from build123d import *

# Parameters (mm, degrees)
BOSS_EXTRUDE1_DEPTH   = 2
F_4_0MM_DOWEL_HOLE1_D = 4


with BuildPart() as part:
    # Sketch1 → Boss-Extrude1 (new body)
    with BuildSketch(Plane(origin=(0, 0, 0), x_dir=(1, 0, 0), z_dir=(0, 1, 0))):
        Polygon((-53.970588235, 35.110294118), (-41.470588235, 35.110294118), (-41.470588235, 47.610294118), (23.529411765, 47.610294118), (23.529411765, 35.110294118), (36.029411765, 35.110294118), (36.029411765, -29.889705882), (23.529411765, -29.889705882), (23.529411765, -42.389705882), (-41.470588235, -42.389705882), (-41.470588235, -29.889705882), (-53.970588235, -29.889705882), align=None)
    extrude(amount=BOSS_EXTRUDE1_DEPTH)

    # Ø4.0mm Dowel Hole1 (through all)
    with Locations(Plane(origin=(0, 2, 0), x_dir=(1, 0, 0), z_dir=(0, 1, 0))):
        with Locations((-43.970588235, 25.110294118), (26.029411765, 25.110294118), (-43.970588235, -19.889705882), (26.029411765, -19.889705882)):
            Hole(F_4_0MM_DOWEL_HOLE1_D / 2)


solid = part.part
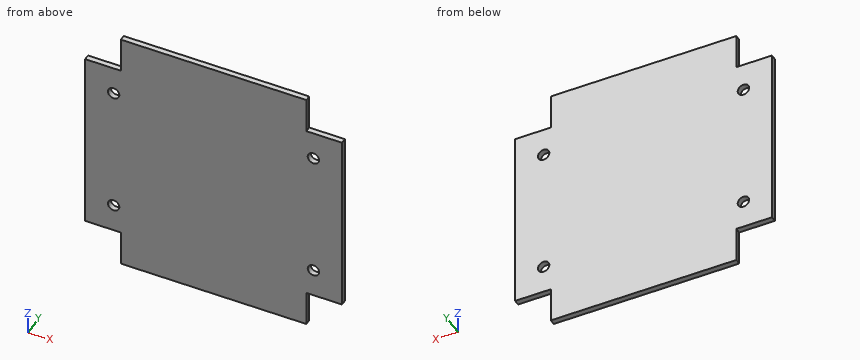
Part model, mm, in its own coordinate system. Coordinates: 2 decimals unless noted, no trailing zeros. Loops run counter-clockwise (first coordinate to the right, second up) from the corner with the lowest first, then second, coordinate; pieces in that order, holes last. Notation, with made-up numbers: (-15, 40) - (-10, 40) arc R19 cw to (-10, 72) - close; hole circle Ø1 at (65.25, 56). An arc over 180 degrees is marked (long way). Write each question's results on one line, items separated by ' | '. Start each with the question number.
Q1. Drop flat-ended pins along their axis: pin 1 Ø0.6 at (y, z) = (1, 33.5) entering from +X; pin 2 Ø0.6 at (y, z) = (1.5, -40) entering from -X; pin 3 Ø0.6 at (x, y) = (31, 1.5) entering from +Z. Give the stop position or say it passes through.
Q2. Slice it at C-C on z = 35. Give the cut face in (x, y).
Q3. Probe line 1 along X through (y, z) = (1.7, -24); line 2 along X through (y, z) = (0.4, -24.5); line 3 along Z through (x, y) = (24.5, 0.7). List the from-to ranges inside material, lowest first.
Q4. Slice it at D-D on x = -48. Give the cut face in (y, z).
Q5. Slice it at A-A on x = 27. Give the cut face in (y, z), and give its area (3 significant figures).
Q6. Slice it at B-B on y = 1.55. Give the cut face in (x, z).
Answer:
1) pin 1: stops at x = 23.53 | pin 2: stops at x = -41.47 | pin 3: stops at z = 29.89
2) outline: (-41.47, 0) - (23.53, 0) - (23.53, 2) - (-41.47, 2) - close
3) line 1: x = -53.97 to -45.63, -42.31 to 24.37, 27.69 to 36.03 | line 2: x = -53.97 to -45.88, -42.07 to 24.12, 27.93 to 36.03 | line 3: z = -35.11 to -26.4, -23.82 to 18.6, 21.18 to 29.89
4) outline: (0, -35.11) - (2, -35.11) - (2, 29.89) - (0, 29.89) - close
5) outline: (0, -35.11) - (2, -35.11) - (2, -26.86) - (0, -26.86) - close; (0, -23.36) - (2, -23.36) - (2, 18.14) - (0, 18.14) - close; (0, 21.64) - (2, 21.64) - (2, 29.89) - (0, 29.89) - close | area: 116 mm2
6) outline: (-53.97, -35.11) - (-41.47, -35.11) - (-41.47, -47.61) - (23.53, -47.61) - (23.53, -35.11) - (36.03, -35.11) - (36.03, 29.89) - (23.53, 29.89) - (23.53, 42.39) - (-41.47, 42.39) - (-41.47, 29.89) - (-53.97, 29.89) - close; hole circle Ø4 at (-43.97, -25.11); hole circle Ø4 at (-43.97, 19.89); hole circle Ø4 at (26.03, -25.11); hole circle Ø4 at (26.03, 19.89)
